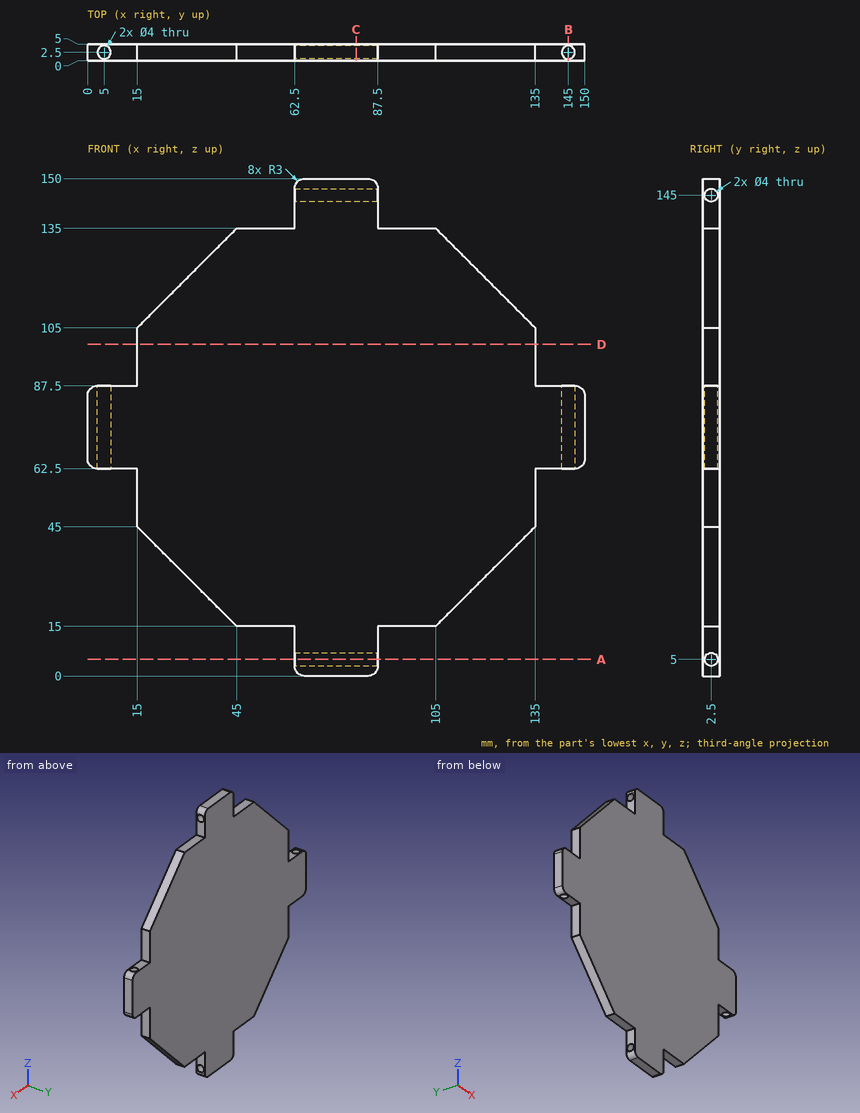
Geometry check sheet. Reference: drawing and pictorial views, mm from the part's lowest x, y, z. Round coordinates to 2 decimals unless told otherwise and drop trailing zeros. Write each loop counter-clockwise with the first axis right and the second up, starting at its lowest first coordinate (ties: lowest second). Pieces come first, ordered by that corner, then holes. Notation, with made-up numbers: (-31, -25) -> (12, -25) arc R23 ccw to (12, -8) -> close; hole circle Ø1 at (30.25, 28.25). An arc over 180 degrees is marked (long way). Put each result on its own line as item: value.
1) Cross-section at B-B, the plane x = 145. Enter the section's corners in (y, z).
Recorded:
outline: (0, 62.5) -> (0.5, 62.5) -> (0.5, 87.5) -> (0, 87.5) -> close; (4.5, 62.5) -> (5, 62.5) -> (5, 87.5) -> (4.5, 87.5) -> close
2) Cross-section at D-D, the plane z = 100. Enter the section's corners in (x, y).
Recorded:
outline: (15, 0) -> (135, 0) -> (135, 5) -> (15, 5) -> close
3) Cross-section at A-A, the plane z = 5. Enter the section's corners in (x, y).
Recorded:
outline: (62.5, 0) -> (87.5, 0) -> (87.5, 0.5) -> (62.5, 0.5) -> close; (62.5, 4.5) -> (87.5, 4.5) -> (87.5, 5) -> (62.5, 5) -> close
4) Depth check by flat-ended pin: P1, Ø1.5, axis at y = 3.5, z = 55, coming from the -X side; P2, Ø4, axis at x = 71.5, z = 100, coming from the -Y side; P3, Ø1.5, axis at x = 98.5, y = 2, coming from the +Z side; P4, Ø1.5, axis at y = 2, z = 140.5, coming from the -X side. Enter the tip coordinate at first touch or a pass-through.
Recorded:
P1: stops at x = 15
P2: stops at y = 0
P3: stops at z = 135
P4: stops at x = 62.5
5) Cross-section at C-C, the plane x = 81. Enter the section's corners in (y, z), plus the area to 3 significant figures.
Recorded:
outline: (0, 0) -> (5, 0) -> (5, 150) -> (0, 150) -> close; hole circle Ø4 at (2.5, 5); hole circle Ø4 at (2.5, 145)
area: 725 mm2
6) Thickness scan on probe 1 along Z at (x, y) = (69, 2.2); probe 2 along X at (y, z) = (1.7, 74); probe 3 along X at (y, z) = (4.2, 81). Record the ranges inside material, lowest first. Write a range as from..to.
Recorded:
probe 1: z = 0..3.02, 6.98..143.02, 146.98..150
probe 2: x = 0..3.17, 6.83..143.17, 146.83..150
probe 3: x = 0..3.95, 6.05..143.95, 146.05..150
